from build123d import *

# Parameters (mm, degrees)
SKETCH1_R           = 11.5
BOSS_EXTRUDE1_DEPTH = 13
SKETCH2_R           = 10
BOSS_EXTRUDE2_DEPTH = 5
SKETCH3_R           = 11.5
BOSS_EXTRUDE3_DEPTH = 13
SKETCH4_R           = 10
BOSS_EXTRUDE4_DEPTH = 5
SKETCH5_R           = 11.5
BOSS_EXTRUDE5_DEPTH = 13
SKETCH6_R           = 10
BOSS_EXTRUDE6_DEPTH = 5
SKETCH7_R           = 11.5
BOSS_EXTRUDE7_DEPTH = 13
SKETCH8_R           = 5
CUT_EXTRUDE1_DEPTH  = 68


with BuildPart() as part:
    # Sketch1 → Boss-Extrude1 (new body)
    with BuildSketch(Plane.XY):
        Circle(SKETCH1_R)
    extrude(amount=BOSS_EXTRUDE1_DEPTH)

    # Sketch2 → Boss-Extrude2 (add)
    with BuildSketch(Plane.XY.offset(13)):
        Circle(SKETCH2_R)
    extrude(amount=BOSS_EXTRUDE2_DEPTH)

    # Sketch3 → Boss-Extrude3 (add)
    with BuildSketch(Plane.XY.offset(18)):
        Circle(SKETCH3_R)
    extrude(amount=BOSS_EXTRUDE3_DEPTH)

    # Sketch4 → Boss-Extrude4 (add)
    with BuildSketch(Plane.XY.offset(31)):
        Circle(SKETCH4_R)
    extrude(amount=BOSS_EXTRUDE4_DEPTH)

    # Sketch5 → Boss-Extrude5 (add)
    with BuildSketch(Plane.XY.offset(36)):
        Circle(SKETCH5_R)
    extrude(amount=BOSS_EXTRUDE5_DEPTH)

    # Sketch6 → Boss-Extrude6 (add)
    with BuildSketch(Plane.XY.offset(49)):
        Circle(SKETCH6_R)
    extrude(amount=BOSS_EXTRUDE6_DEPTH)

    # Sketch7 → Boss-Extrude7 (add)
    with BuildSketch(Plane.XY.offset(54)):
        Circle(SKETCH7_R)
    extrude(amount=BOSS_EXTRUDE7_DEPTH)

    # Sketch8 → Cut-Extrude1 (cut, through all)
    with BuildSketch(Plane.XY.offset(67)):
        Circle(SKETCH8_R)
    extrude(amount=-CUT_EXTRUDE1_DEPTH, mode=Mode.SUBTRACT)


solid = part.part
Here's how the part is built. I have some questions about the finished solid (model axes, mm). A direction names the side the tool comes from. Round coordinates to 2 decimals unless told otherwise and drop trailing zeros. Order: outer loops, then holes, each group sorted by start corner. A loop starts at its lowest first (then second) coordinate and runs counter-clockwise, first axis right, second up. Notation, with made-up numbers: M 32.5,70.25 L 89.5,70.25 A11 cw 89.5,78.25 Z; hole C 55.5,53.5 d3. An arc over 180 degrees is marked long. Return JSON: item names as keys, results as strings. Group by question number.
1. If we mould it in two halves opening along Y, with no side actions, what happens to faces 1 (the face through (-1.5, 11.4, 6.4)), 2 (the face through (-9, 5, 13)), 3 (the face through (-1.08, -4.88, 33.97))? For each: pulls with the +Y half, pulls with the -Y half, needs draft (parallel to the pull), parting line crosses it, or undercut.
2. I'm going to push flat-ended pins straight in: pin 1 Ø12 at (y, z) = (-8, 50) entering from -X; pin 2 Ø11.5 at (x, y) = (-1, 2.5) entering from -Z; pin 3 Ø1 at (x, z) = (-7, 34) entering from -Y; pin 4 Ø1 at (y, z) = (-2.5, 32.5) entering from +X. Where does each tip first touch, or does it pass through?
3. On a 3-axis mill with a long thin cutter (end or side, diameter ignored), from which of +Z, -Z, +X, -X, +Y, -Y can I reach the whole of each face in a straight line? I mean faces 4 (the face through (-2.17, -9.76, 15.46)), 5 (the face through (-1.5, 11.4, 60.4)). Say none if no direction works.
4. If we section it at C-C on z = 42.5: List the corners of the cut face in (x, y) for me, then the cut area to 3 significant figures.
5. If we section it at D-D on x = 8.5: List the corners of the cut face in (y, z) for me.
6. Please list where these lines run through material, in increasing order: probe 1 along Z at (x, y) = (10.5, 0.75); probe 2 along Y at (x, z) = (0, 21); probe 3 along Y at (x, z) = (0, 52).
Reply:
{
 "1": {"face 1": "parting line crosses it", "face 2": "needs draft", "face 3": "undercut"},
 "2": {"pin 1": "x = -11.31", "pin 2": "z = 0", "pin 3": "y = -7.6", "pin 4": "x = 9.8"},
 "3": {"face 4": "none", "face 5": "+Z, -Z"},
 "4": {"outline": "C 0,0 d23; hole C 0,0 d10", "area": "337 mm^2"},
 "5": {"outline": "M -7.75,0 L 7.75,0 L 7.75,13 L 5.27,13 L 5.27,18 L 7.75,18 L 7.75,31 L 5.27,31 L 5.27,36 L 7.75,36 L 7.75,49 L 5.27,49 L 5.27,54 L 7.75,54 L 7.75,67 L -7.75,67 L -7.75,54 L -5.27,54 L -5.27,49 L -7.75,49 L -7.75,36 L -5.27,36 L -5.27,31 L -7.75,31 L -7.75,18 L -5.27,18 L -5.27,13 L -7.75,13 Z"},
 "6": {"probe 1": "0 to 13, 18 to 31, 36 to 49, 54 to 67", "probe 2": "-11.5 to -5, 5 to 11.5", "probe 3": "-10 to -5, 5 to 10"}
}
